from build123d import *

# Parameters (mm, degrees)
SCHIZZO1_W                     = 90
SCHIZZO1_H                     = 100
BASE_FLANGIA1_DEPTH            = 3
BORDO_FLANGIA1_STRIP_W         = 18
BORDO_FLANGIA1_STRIP_H         = 3
BORDO_FLANGIA1_STRIP_CUT_DEPTH = 90
BORDO_FLANGIA1_DEPTH           = 90
RACCORDO1_R                    = 10
SCHIZZO10_R                    = 4.5
TAGLIO_ESTRUSIONE1_DEPTH       = 10
SCHIZZO9_R                     = 12
TAGLIO_ESTRUSIONE2_DEPTH       = 10
SCHIZZO11_W                    = 90
SCHIZZO11_H                    = 58
TAGLIO_ESTRUSIONE3_DEPTH       = 10
SCHIZZO12_W                    = 90
SCHIZZO12_H                    = 15
TAGLIO_ESTRUSIONE4_DEPTH       = 10
FORO_START                     = -103
FORO_PER_VITE_M4_1_OUTLINE_R   = 2.25
FORO_PER_VITE_M4_1_DEPTH       = 3


# Read off the part's stored shape, not the designer's step: Foro per Vite M4-1
# Sheet-metal steps are written as plain solids
with BuildPart() as part:
    # Schizzo1 → Base-Flangia1 (new body)
    with BuildSketch(Plane(origin=(0, 0, 0), x_dir=(1, 0, 0), z_dir=(0, 1, 0))):
        with Locations((-45, 50)):
            Rectangle(SCHIZZO1_W, SCHIZZO1_H)
    extrude(amount=-BASE_FLANGIA1_DEPTH)

    # Bordo-Flangia1 strip (across the edge) → Bordo-Flangia1 strip cut (cut)
    with BuildSketch(Plane(origin=(0, 0, -100), x_dir=(0, 0, 1), z_dir=(-1, 0, 0))):
        with Locations((-6, -1.5)):
            Rectangle(BORDO_FLANGIA1_STRIP_W, BORDO_FLANGIA1_STRIP_H)
    extrude(amount=BORDO_FLANGIA1_STRIP_CUT_DEPTH, mode=Mode.SUBTRACT)

    # Bordo-Flangia1 section (across the edge) → Bordo-Flangia1 (add)
    with BuildSketch(Plane(origin=(0, 0, -100), x_dir=(0, 0, 1), z_dir=(-1, 0, 0))):
        with BuildLine():
            Line((-3, 3), (-3, 100))
            Line((-3, 100), (0, 100))
            Line((0, 100), (0, 3))
            ThreePointArc((0, 3), (0.878679656, 0.878679656), (3, 0))
            Line((3, 0), (3, -3))
            ThreePointArc((3, -3), (-1.242640687, -1.242640687), (-3, 3))
        make_face()
    extrude(amount=BORDO_FLANGIA1_DEPTH)

    # Raccordo1
    raccordo1_edges = [part.edges().sort_by_distance(p)[0] for p in [
        (0, 100, -101.5),
        (-90, 100, -101.5),
        (0, -1.5, 0),
        (-90, -1.5, 0),
    ]]
    fillet(raccordo1_edges, radius=RACCORDO1_R)

    # Schizzo10 → Taglio-Estrusione1 (cut)
    with BuildSketch(Plane.XZ.offset(3)):
        with Locations(Location((-60.5, -89.5, 0), (0, 0, 270))):
            Circle(SCHIZZO10_R)
        with Locations(Location((-60.5, -65.5, 0), (0, 0, 270))):
            Circle(SCHIZZO10_R)
        with Locations(Location((-29.5, -65.5, 0), (0, 0, 270))):
            Circle(SCHIZZO10_R)
        with Locations(Location((-29.5, -89.5, 0), (0, 0, 270))):
            Circle(SCHIZZO10_R)
    extrude(amount=-TAGLIO_ESTRUSIONE1_DEPTH, mode=Mode.SUBTRACT)

    # Schizzo9 → Taglio-Estrusione2 (cut)
    with BuildSketch(Plane.XY.offset(-100)):
        with Locations(Location((-45, 15, 0), (0, 0, 270))):
            Circle(SCHIZZO9_R)
    extrude(amount=-TAGLIO_ESTRUSIONE2_DEPTH, mode=Mode.SUBTRACT)

    # Schizzo11 → Taglio-Estrusione3 (cut)
    with BuildSketch(Plane(origin=(0, 0, 0), x_dir=(1, 0, 0), z_dir=(0, 1, 0))):
        with Locations((-45, 29)):
            Rectangle(SCHIZZO11_W, SCHIZZO11_H)
    extrude(amount=-TAGLIO_ESTRUSIONE3_DEPTH, mode=Mode.SUBTRACT)

    # Schizzo12 → Taglio-Estrusione4 (cut)
    with BuildSketch(Plane.XY.offset(-100)):
        with Locations((-45, 92.5)):
            Rectangle(SCHIZZO12_W, SCHIZZO12_H)
    extrude(amount=-TAGLIO_ESTRUSIONE4_DEPTH, mode=Mode.SUBTRACT)

    # Foro per Vite M4-1 outline → Foro per Vite M4-1 (cut)
    with BuildSketch(Plane.XY.offset(FORO_START)):
        with Locations((-10, 74)):
            Circle(FORO_PER_VITE_M4_1_OUTLINE_R)
        with Locations((-80, 14)):
            Circle(FORO_PER_VITE_M4_1_OUTLINE_R)
        with Locations((-10, 14)):
            Circle(FORO_PER_VITE_M4_1_OUTLINE_R)
        with Locations((-80, 74)):
            Circle(FORO_PER_VITE_M4_1_OUTLINE_R)
    extrude(amount=FORO_PER_VITE_M4_1_DEPTH, mode=Mode.SUBTRACT)


solid = part.part
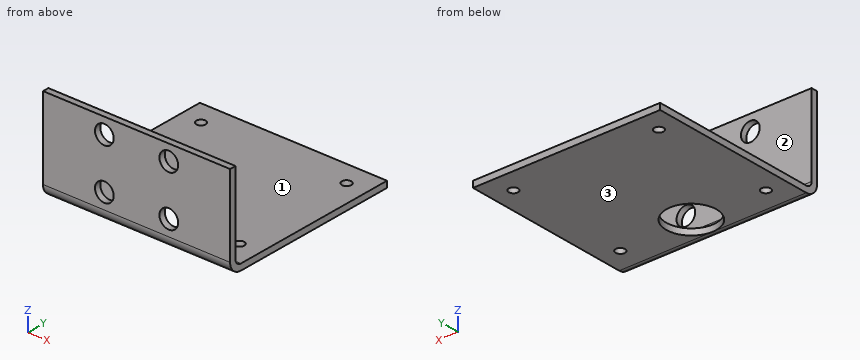
For this review, take the finished solid that the model builds, in its own axes (mm). Face numbers are marked on the shaded views. Round coordinates to 2 decimals unless told otherwise and drop trailing zeros. Write each loop counter-clockwise with the first axis right and the second up, starting at its lowest first coordinate (ties: lowest second). Pieces come first, ordered by that corner, then holes. Notation, with made-up numbers: (63, 65.25) - (95, 65.25) arc R9 cw to (95, 81.25) - close; hole circle Ø3 at (-4, 31.5). An arc over 180 degrees is marked (long way). Write item = value, one per line. Start each with the question number.
1. Draft analysis for pull direction Z (two halves, no side actions). For the marked faces 1, 2 and 3, state which applies: released by +Z, released by -Z, zero draft, split by the parting line, or undercut.
2. Wall thickness on L1, parallel to Y at x = -10, z = -100.55; L2, parallel to Y at x = -80, z = -100.85; L3, parallel to Y at x = -84, z = -66: over which ranges is each line inside the solid? List them lowest first.
3. Consider section C-C on z = -89.5. State the section outline as (x, y) points.
4. Consider section A-A on x = -10. State the section outline as (y, z) points.
5. Consider section B-B on y = 74. State the section outline as (x, z) points, plus the area to 3 significant figures.
6. Consider section D-D on y = 14. State the section outline as (x, z) points, plus the area to 3 significant figures.
7. For pin 1 Ø2 at (x, z) = (-75.5, -64) entering from +Y; pin 2 Ø6 at (x, y) = (-75.5, 35) entering from +Z; pin 3 Ø12 at (y, z) = (14.5, -89.5) entering from +X, all flat-tipped, find the tip position at first contact; note any pin that passes through.
Evaluation:
q1.face_1 = released by +Z
q1.face_2 = zero draft
q1.face_3 = released by -Z
q2.L1 = -1.84 to 11.75, 16.25 to 71.75, 76.25 to 85
q2.L2 = -1.6 to 11.75, 16.25 to 71.75, 76.25 to 85
q2.L3 = -3 to 0
q3.outline = (-90, -3) - (-65, -3) - (-65, 0) - (-90, 0) - close; (-56, -3) - (-34, -3) - (-34, 0) - (-56, 0) - close; (-25, -3) - (0, -3) - (0, 0) - (-25, 0) - close
q4.outline = (-3, -97) arc R6 ccw to (3, -103) - (11.75, -103) - (11.75, -100) - (3, -100) arc R3 cw to (0, -97) - (0, -58) - (-3, -58) - close; (16.25, -103) - (71.75, -103) - (71.75, -100) - (16.25, -100) - close; (76.25, -103) - (85, -103) - (85, -100) - (76.25, -100) - close
q5.outline = (-90, -103) - (-82.25, -103) - (-82.25, -100) - (-90, -100) - close; (-77.75, -103) - (-12.25, -103) - (-12.25, -100) - (-77.75, -100) - close; (-7.75, -103) - (0, -103) - (0, -100) - (-7.75, -100) - close
q5.area = 243 mm2
q6.outline = (-90, -103) - (-82.25, -103) - (-82.25, -100) - (-90, -100) - close; (-77.75, -103) - (-56.96, -103) - (-56.96, -100) - (-77.75, -100) - close; (-33.04, -103) - (-12.25, -103) - (-12.25, -100) - (-33.04, -100) - close; (-7.75, -103) - (0, -103) - (0, -100) - (-7.75, -100) - close
q6.area = 171 mm2
q7.pin_1 = 0
q7.pin_2 = -100
q7.pin_3 = through
